Autodesk Fusion 360 part; units mm, degrees
sketch "Sketch1" plane through (0, 0, 0) normal (0, 1, 0) x (1, 0, 0)
  line L0 (0, 0) -> (4.5, 0)
  line L1 (4.5, 0) -> (4.5, -4.5)
  line L2 (4.5, -4.5) -> (0, -4.5)
  line L3 (0, -4.5) -> (0, 0)
  line L4 (0, -4.5) -> (4.5, 0) construction
  line L5 (4.5, -4.5) -> (0, 0) construction
  circle A0 centre (2.25, -2.25) radius 4
  line L6 (4.5, -2.25) -> (4.5, -1.75)
  line L7 (4.5, -1.75) -> (5, -1.75)
  line L8 (5, -1.75) -> (5, -2.75)
  line L9 (5, -2.75) -> (4.5, -2.75)
  line L10 (0, -2.75) -> (-0.5, -2.75)
  line L11 (-0.5, -2.75) -> (-0.5, -1.75)
  line L12 (-0.5, -1.75) -> (0, -1.75)
  line L13 (2.25, -2.25) -> (2.25, -4.5) construction
  line L14 (2.25, -2.25) -> (2.25, 0) construction
  line L15 (2.25, -4.5) -> (2.75, -4.5) construction
  line L16 (2.75, -4.5) -> (2.75, -5)
  line L17 (2.75, -5) -> (1.75, -5)
  line L18 (1.75, -5) -> (1.75, -4.5)
  line L19 (2.25, 0) -> (2.75, 0) construction
  line L20 (2.75, 0) -> (2.75, 0.5)
  line L21 (2.75, 0.5) -> (1.75, 0.5)
  line L22 (1.75, 0.5) -> (1.75, 0)
  dimension "d1" = 4.5
  dimension "d2" = 4.5
  dimension "d3" = 4.5
  dimension "d4" = 8
  dimension "d5" = 0.5
  dimension "d6" = 1
  dimension "d7" = 0.5
  dimension "d8" = 1
  dimension "d9" = 0.5
  dimension "d10" = 0.5
  dimension "d11" = 1
  dimension "d12" = 0.5
  dimension "d13" = 0.5
  dimension "d14" = 1
extrude "Extrude1" add sketch "Sketch1" along normal blind 2
sketch "Sketch2" plane through (0, 0, 0) normal (0, -1, 0) x (1, 0, 0)
  line L0 (2.75, 0) -> (2.75, -0.5)
  line L1 (2.75, -0.5) -> (1.75, -0.5)
  line L2 (1.75, -0.5) -> (1.75, 0)
  line L3 (1.75, 0) -> (0, 0)
  line L4 (0, 0) -> (0, 1.75)
  line L5 (0, 1.75) -> (-0.5, 1.75)
  line L6 (-0.5, 1.75) -> (-0.5, 2.75)
  line L7 (-0.5, 2.75) -> (0, 2.75)
  line L8 (0, 2.75) -> (0, 4.5)
  line L9 (0, 4.5) -> (1.75, 4.5)
  line L10 (1.75, 4.5) -> (1.75, 5)
  line L11 (1.75, 5) -> (2.75, 5)
  line L12 (2.75, 5) -> (2.75, 4.5)
  line L13 (2.75, 4.5) -> (4.5, 4.5)
  line L14 (4.5, 4.5) -> (4.5, 2.75)
  line L15 (4.5, 2.75) -> (5, 2.75)
  line L16 (5, 2.75) -> (5, 1.75)
  line L17 (5, 1.75) -> (4.5, 1.75)
  line L18 (4.5, 1.75) -> (4.5, 0)
  line L19 (4.5, 0) -> (2.75, 0)
  circle A0 centre (2.25, 2.25) radius 4
extrude "Extrude2" add sketch "Sketch2" along normal blind 2 contours L0 L1 L2 L3 L4 L5 L6 L7 L8 L9 L10 L11 L12 L13 L14 L15 L16 L17 L18 L19 | A0
sketch "Sketch3" plane through (0, -2, 0) normal (0, -1, 0) x (1, 0, 0)
  circle A0 centre (2.25, 2.25) radius 4
sketch "Sketch4" plane through (0, -2, 0) normal (0, -1, 0) x (1, 0, 0)
  circle A0 centre (2.25, 2.25) radius 1.25
  point P0 (2.25, 2.25)
  dimension "d19" = 2.5
  dimension "d21" = 0
extrude "Extrude3" add sketch "Sketch4" along normal blind 15
Here's how the part is built. I have some questions about the finished solid (model axes, mm). A direction names the side the tool comes from. Round coordinates to 2 decimals unless told otherwise and drop trailing zeros. Order: outer loops, then holes, each group sorted by start corner. A loop starts at its lowest first (then second) coordinate and runs counter-clockwise, first axis right, second up. Notation, with made-up numbers: M 45,72.5 L 73,72.5 A10 cw 73,82.5 Z; hole C 21,83.25 d1. An arc over 180 degrees is marked long. Answer as CSV lines item,"result".
Item 1: Please list where these lines run through material, in increasing order: L1, parallel to Y at x = 1.75, z = -0.75; L2, parallel to Y at x = 1.75, z = 1; L3, parallel to Z at x = -0.25, y = 0.75. Write a range as [from, to].
From the geometry:
L1,"[-2, 2]"
L2,"[-2, 0]"
L3,"[-0.87, 1.75], [2.75, 5.37]"
Item 2: Which directions (+Z, -Z, +X, -X, +Y, -Y) give clear straight access to the entire face, cutting with the end or side of a thin tool? Please do faces 4 (the cylindrical face through (5.945, -0.028, 0.718)), 5 (the flat face through (1, -2, 1)), 6 (the flat face through (2, 1, 5)).
From the geometry:
face 4,"+Y, -Y"
face 5,"-Y"
face 6,"+Y"
Item 3: Imagine slicing it at D-D on x = 4. List the corners of the cut face in (y, z) for me.
From the geometry:
outline,"M -2,-1.35 L 2,-1.35 L 2,0 L 0,0 L 0,4.5 L 2,4.5 L 2,5.85 L -2,5.85 Z"
Item 4: Imagine slicing it at C-C on y = -8.75. List the corners of the cut face in (x, z) for me.
From the geometry:
outline,"C 2.25,2.25 d2.5"
Item 5: For pin 1 (3 mm diameter, centred on x = 1.5, y = -10.5, fed in from -Z); pin 2 (2 mm diameter, centred on x = 0.5, y = -14, fed in from +Z); pin 3 (1 mm diameter, centred on y = -13.5, z = 3, fed in from -X), each with a flat end and sliding along its axis, tell me the tip position at first contact or that it passes through.
From the geometry:
pin 1,"z = 1"
pin 2,"z = 3.25"
pin 3,"x = 1.03"
Item 6: Imagine slicing it at A-A on x = 2.25. List the corners of the cut face in (y, z) for me.
From the geometry:
outline,"M -17,1 L -2,1 L -2,-1.75 L 2,-1.75 L 2,-0.5 L 0,-0.5 L 0,5 L 2,5 L 2,6.25 L -2,6.25 L -2,3.5 L -17,3.5 Z"
Item 7: We'd pull the mould along Z, two halves only. Please class faces 1 (the cylindrical face through (3.44, -9.4, 1.87)), 2 (the flat face through (1, 1, 4.5)), 3 (the flat face through (2, -17, 2)): +Z half, -Z half, draft (parallel to the pull), parting line (faces both ways), or undercut.
From the geometry:
face 1,"parting line"
face 2,"undercut"
face 3,"draft"
Item 8: Imagine slicing it at B-B on z = 2.25. List the corners of the cut face in (x, y) for me.
From the geometry:
outline,"M -1.75,-2 L 1,-2 L 1,-17 L 3.5,-17 L 3.5,-2 L 6.25,-2 L 6.25,2 L 5,2 L 5,0 L -0.5,0 L -0.5,2 L -1.75,2 Z"
